Work out the finished part from the listing and answer in its coordinate system (mm). Face numbers are marked on the shaded views. A direction names the side the tool comes from. Give positions to 0.01 mm unless a question says otherwise; leave off trailing zeros. Loops run counter-clockwise (first coordinate to the right, second up) from the corner with the lowest first, then second, coordinate; pieces in that order, holes last. Notation, with made-up numbers: M 8,69.25 L 34,69.25 A27 ccw 34,96.25 Z; hole C -11,-20 d7. An arc over 180 degrees is marked long. Use a Markdown table: item, result.
```python
from build123d import *

# Parameters (mm, degrees)
BOSS_EXTRUDE1_DEPTH  = 0.21
SKETCH2_W            = 4
SKETCH2_H            = 0.21
CUT_EXTRUDE1_DEPTH   = 2.6
SWEEP1_START         = 0.285
SWEEP1_DEPTH         = 1.715
FILLET1_START        = -3
FILLET1_DEPTH        = 6
FILLET1_START_2      = -2
FILLET1_2_DEPTH      = 1.715
FILLET1_START_3      = 0.285
FILLET1_3_DEPTH      = 1.715
SKETCH4_R            = 0.25
CUT_EXTRUDE2_DEPTH   = 0.15
FILLET2_R            = 0.25
FILLET3_R            = 0.2
FILLET2_OF_MIRROR4_R = 0.25
FILLET3_OF_MIRROR4_R = 0.2
SKETCH6_W            = 4
SKETCH6_H            = 0.209488451
CUT_EXTRUDE5_DEPTH   = 15.914789915


with BuildPart() as part:
    # Sketch1 → Boss-Extrude1 (new body)
    with BuildSketch(Plane.XY):
        with BuildLine():
            Line((-0.285, 7.215), (-2, 7.215))
            Line((-2, 7.215), (-2, -1.085))
            Line((-2, -1.085), (-0.46, -2.485))
            Line((-0.46, -2.485), (-0.46, -5.985))
            Line((-0.46, -5.985), (-0.1, -7.585))
            Line((-0.1, -7.585), (0.1, -7.585))
            Line((0.1, -7.585), (0.46, -5.985))
            Line((0.46, -5.985), (0.46, -2.485))
            Line((0.46, -2.485), (2, -1.085))
            Line((2, -1.085), (2, 7.215))
            Line((2, 7.215), (0.285, 7.215))
            Line((0.285, 7.215), (0.285, 0))
            ThreePointArc((0.285, 0), (0, -0.285), (-0.285, 0))
            Line((-0.285, 0), (-0.285, 7.215))
        make_face()
    extrude(amount=BOSS_EXTRUDE1_DEPTH)

    # Sketch2 → Cut-Extrude1 (cut)
    with BuildSketch(Plane(origin=(0, 7.215, 0), x_dir=(1, 0, 0), z_dir=(0, 1, 0))):
        with Locations((0, -0.105)):
            Rectangle(SKETCH2_W, SKETCH2_H)
    extrude(amount=-CUT_EXTRUDE1_DEPTH, mode=Mode.SUBTRACT)

    # Sweep1: read off the stored shape, not the designer's step
    # Sweep1 outline → Sweep1 (add)
    with BuildSketch(Plane.YZ.offset(SWEEP1_START)):
        Polygon((4.615, 0), (7.215, -0.181809711), (7.215, 0.028190289), (4.615, 0.21), align=None)
    extrude(amount=SWEEP1_DEPTH)

    # Mirror3: part across plane


with BuildPart() as part_1:
    add(part.part)
    add(part.part.mirror(Plane(origin=(0, 0, 0), x_dir=(0, 0, 1), z_dir=(1, 0, 0))))

    # Fillet1: read off the stored shape, not the designer's step
    # Fillet1 outline → Fillet1 (cut)
    with BuildSketch(Plane.YZ.offset(FILLET1_START)):
        with BuildLine():
            ThreePointArc((4.475316922, 0.21), (4.614914909, 0.207563308), (4.754342817, 0.200256201))
            Line((4.754342817, 0.200256201), (4.615, 0.21))
            Line((4.615, 0.21), (4.475316922, 0.21))
        make_face()
    extrude(amount=FILLET1_DEPTH, mode=Mode.SUBTRACT)

    # Fillet1 2 outline → Fillet1 2 (add)
    with BuildSketch(Plane.YZ.offset(FILLET1_START_2)):
        with BuildLine():
            Line((4.615, 0), (4.475316922, 0))
            ThreePointArc((4.475316922, 0), (4.614914909, -0.002436692), (4.754342817, -0.009743799))
            Line((4.754342817, -0.009743799), (4.615, 0))
        make_face()
    extrude(amount=FILLET1_2_DEPTH)

    # Fillet1 3 outline → Fillet1 3 (add)
    with BuildSketch(Plane.YZ.offset(FILLET1_START_3)):
        with BuildLine():
            Line((4.615, 0), (4.475316922, 0))
            ThreePointArc((4.475316922, 0), (4.614914909, -0.002436692), (4.754342817, -0.009743799))
            Line((4.754342817, -0.009743799), (4.615, 0))
        make_face()
    extrude(amount=FILLET1_3_DEPTH)

    # Sketch4 → Cut-Extrude2 (cut)
    with BuildSketch(Plane(origin=(0, 0.022456431, 0.32114193), x_dir=(-1, 0, 0), z_dir=(0, -0.06975647374412543, -0.9975640502598243))):
        with Locations(Location((-1.1425, 6.260107027, 0), (0, 0, 90))):
            Circle(SKETCH4_R)
        with Locations(Location((-1.1425, 5.260107027, 0), (0, 0, 90))):
            Circle(SKETCH4_R)
    cut_extrude2 = extrude(amount=-CUT_EXTRUDE2_DEPTH, mode=Mode.SUBTRACT)

    # Fillet2
    # the kernel refuses this fillet: 0.25 mm, written as the material it adds along each edge
    with BuildSketch(Plane(origin=(1.1425, 6.277777623, 0.034093547), x_dir=(0, 0.9975640502598242, -0.06975647374412533), z_dir=(-1, 0, 0))) as fillet2_piece_1:
        with BuildLine():
            CenterArc((0.020871215, 0.25), FILLET2_R, 270, 66.421821522)
            Line((0.020871215, 0), (0.020871215, -0.005))
            Line((0.020871215, -0.005), (0.25, -0.005))
            Line((0.25, -0.005), (0.255, 0))
            ThreePointArc((0.255, 0), (0.255, 0.075), (0.254582576, 0.148))
            Line((0.254582576, 0.148), (0.25, 0.15))
        make_face()
    revolve(axis=Axis((1.1425, 6.277777623, 0.034093547), (0, -0.06975647374412543, -0.9975640502598243)))
    with BuildSketch(Plane(origin=(1.1425, 5.280213573, 0.10385002), x_dir=(0, 0.9975640502598242, -0.06975647374412533), z_dir=(-1, 0, 0))) as fillet2_piece_2:
        with BuildLine():
            CenterArc((0.020871215, 0.25), FILLET2_R, 270, 66.421821522)
            Line((0.020871215, 0), (0.020871215, -0.005))
            Line((0.020871215, -0.005), (0.25, -0.005))
            Line((0.25, -0.005), (0.255, 0))
            ThreePointArc((0.255, 0), (0.255, 0.075), (0.254582576, 0.148))
            Line((0.254582576, 0.148), (0.25, 0.15))
        make_face()
    revolve(axis=Axis((1.1425, 5.280213573, 0.10385002), (0, -0.06975647374412543, -0.9975640502598243)))

    # Fillet3
    fillet3_edges = [part_1.edges().sort_by_distance(p)[0] for p in [
        (1.1425, 6.01792314, -0.098101943),
        (1.1425, 5.020359089, -0.028345469),
    ]]
    fillet(fillet3_edges, radius=FILLET3_R)

    # Mirror4: Cut-Extrude2 across plane
    add(cut_extrude2.mirror(Plane(origin=(0, 0, 0), x_dir=(0, 0, 1), z_dir=(1, 0, 0))), mode=Mode.SUBTRACT)

    # Fillet2 of Mirror4
    # the kernel refuses this fillet: 0.25 mm, written as the material it adds along each edge
    with BuildSketch(Plane(origin=(-1.1425, 6.277777623, 0.034093547), x_dir=(0, 0.9975640502598242, -0.06975647374412533), z_dir=(1, 0, 0))) as fillet2_of_mirror4_piece_1:
        with BuildLine():
            CenterArc((0.020871215, -0.25), FILLET2_OF_MIRROR4_R, 23.578178478, 66.421821522)
            Line((0.020871215, 0), (0.020871215, 0.005))
            Line((0.020871215, 0.005), (0.25, 0.005))
            Line((0.25, 0.005), (0.255, 0))
            ThreePointArc((0.255, 0), (0.255, -0.075), (0.254582576, -0.148))
            Line((0.254582576, -0.148), (0.25, -0.15))
        make_face()
    revolve(axis=Axis((-1.1425, 6.277777623, 0.034093547), (0, 0.06975647374412543, 0.9975640502598243)))
    with BuildSketch(Plane(origin=(-1.1425, 5.280213573, 0.10385002), x_dir=(0, 0.9975640502598242, -0.06975647374412533), z_dir=(1, 0, 0))) as fillet2_of_mirror4_piece_2:
        with BuildLine():
            CenterArc((0.020871215, -0.25), FILLET2_OF_MIRROR4_R, 23.578178478, 66.421821522)
            Line((0.020871215, 0), (0.020871215, 0.005))
            Line((0.020871215, 0.005), (0.25, 0.005))
            Line((0.25, 0.005), (0.255, 0))
            ThreePointArc((0.255, 0), (0.255, -0.075), (0.254582576, -0.148))
            Line((0.254582576, -0.148), (0.25, -0.15))
        make_face()
    revolve(axis=Axis((-1.1425, 5.280213573, 0.10385002), (0, 0.06975647374412543, 0.9975640502598243)))

    # Fillet3 of Mirror4
    fillet3_of_mirror4_edges = [part_1.edges().sort_by_distance(p)[0] for p in [
        (-1.1425, 6.01792314, -0.098101943),
        (-1.1425, 5.020359089, -0.028345469),
    ]]
    fillet(fillet3_of_mirror4_edges, radius=FILLET3_OF_MIRROR4_R)

    # Sketch6 → Cut-Extrude5 (cut, through all)
    with BuildSketch(Plane(origin=(0, 7.177930393, -0.501929789), x_dir=(1, 0, 0), z_dir=(-1.513554906801369e-15, -0.9975640502598243, 0.06975647374412539))):
        with Locations((0, 0.426670352)):
            Rectangle(SKETCH6_W, SKETCH6_H)
    extrude(amount=-CUT_EXTRUDE5_DEPTH, mode=Mode.SUBTRACT)


solid = part_1.part
```
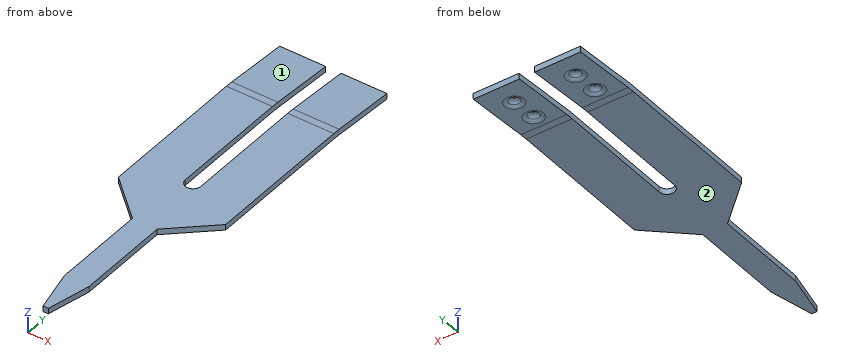
(1) Consider probe 1 along X at (y, z) = (2.5, 0.05) (3 decimals); probe 2 along X at (y, z) = (-5.5, 0.15); probe 3 along Z at (x, y) = (0.35, 4). Determine where each line is inside the solid, lowest interval first. Write a range as [from, to].
Entries:
| item | result |
|---|---|
| probe 1 | x = [-2, -0.285], [0.285, 2] |
| probe 2 | x = [-0.46, 0.46] |
| probe 3 | z = [0, 0.21] |
(2) Which of the six approach directions +Z, -Z, +X, -X, +Y, -Y give full straight-line access (tool end or side, diameter ignored) to the marked faces 1 and 2?
Entries:
| item | result |
|---|---|
| face 1 | +Z, +X, -X, +Y |
| face 2 | -Z, +X, -X, -Y |
(3) A cutting plane is placed at B-B (y = -3). Write down the section's boundary in (x, z).
Entries:
| item | result |
|---|---|
| outline | M -0.46,0 L 0.46,0 L 0.46,0.21 L -0.46,0.21 Z |
(4) Given P1, Ø1.2, axis at x = -0.5, y = -4, coming from the -Z side; P2, Ø1.5, axis at x = -0.5, y = -4.5, coming from the +Z side, each flat-ended and moving along its own axis, determine where each tip first touches the part or whether it passes through.
Entries:
| item | result |
|---|---|
| P1 | stops at z = 0 |
| P2 | stops at z = 0.21 |
(5) A cutting plane is placed at A-A (y = 1.75). Write down the section's boundary in (x, z) (3 decimals).
Entries:
| item | result |
|---|---|
| outline | M -2,0 L -0.285,0 L -0.285,0.21 L -2,0.21 Z; M 0.285,0 L 2,0 L 2,0.21 L 0.285,0.21 Z |
